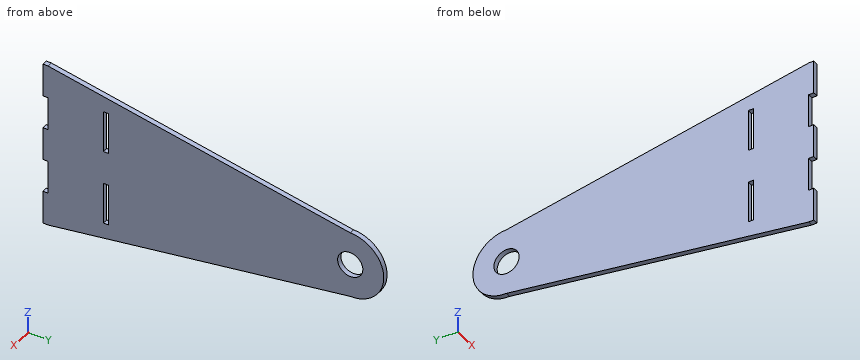
from build123d import *

# Parameters (mm, degrees)
SKETCH2_R           = 7.5
BOSS_EXTRUDE1_DEPTH = 1.5
SKETCH3_W           = 25
SKETCH3_H           = 3
CUT_EXTRUDE1_DEPTH  = 4
SKETCH4_W           = 3
SKETCH4_H           = 20
BOSS_EXTRUDE2_DEPTH = 3


with BuildPart() as part:
    # Sketch2 → Boss-Extrude1 (new, symmetric)
    with BuildSketch(Plane(origin=(0, 0, 0), x_dir=(0, 0, -1), z_dir=(1, 0, 0))):
        with BuildLine():
            Line((50, 0), (-50, 0))
            Line((-50, 0), (-20, 180))
            ThreePointArc((-20, 180), (0, 200), (20, 180))
            Line((20, 180), (50, 0))
        make_face()
        with Locations((0, 180)):
            Circle(SKETCH2_R, mode=Mode.SUBTRACT)
    extrude(amount=BOSS_EXTRUDE1_DEPTH, both=True)

    # Sketch3 → Cut-Extrude1 (cut)
    with BuildSketch(Plane.ZY.offset(1.5)):
        with Locations((22.5, 34.5)):
            Rectangle(SKETCH3_W, SKETCH3_H)
        with Locations((-22.5, 34.5)):
            Rectangle(SKETCH3_W, SKETCH3_H)
    extrude(amount=-CUT_EXTRUDE1_DEPTH, mode=Mode.SUBTRACT)

    # Sketch4 → Boss-Extrude2 (add)
    with BuildSketch(Plane.XZ):
        Rectangle(SKETCH4_W, SKETCH4_H)
        with Locations((0, -40)):
            Rectangle(SKETCH4_W, SKETCH4_H)
        with Locations((0, 40)):
            Rectangle(SKETCH4_W, SKETCH4_H)
    extrude(amount=BOSS_EXTRUDE2_DEPTH)


solid = part.part
Design review of the part built by this model. Coordinates are the model's own, in mm. Round coordinates to 2 decimals unless told otherwise and drop trailing zeros. Write each loop counter-clockwise with the first axis right and the second up, starting at its lowest first coordinate (ties: lowest second). Pieces come first, ordered by that corner, then holes. Notation, with made-up numbers: (46.25, 83.25) - (94.25, 83.25) arc R7 cw to (94.25, 88.25) - close; hole circle Ø1 at (-10.75, -31.75). An arc over 180 degrees is marked (long way). Return JSON: item names as keys, results as strings. Group by question number.
Item 1: We need section A-A on z = 0. Write out the cut boundary in (x, y).
Item 2: Insertion check: P1, Ø0.9, axis at x = 0.5, y = 34, coming from the +Z side; P2, Ø0.9, axis at x = -0.5, y = 34, coming from the -Z side; P3, Ø8, axis at y = 148, z = -29, coming from the -X side; P4, Ø1, axis at x = 0.5, y = 84.5, coming from the +Z side. Each pin has a flat end and moves straight along its axis. Give the tip position at first contact, or say it passes through.
Item 3: We need section B-B on x = 0. Write out the cut boundary in (y, z).
Item 4: We need section D-D on y = 49.5. Write out the cut boundary in (x, z).
Item 5: We need section C-C on z = 32. Write out the cut boundary in (x, y), and give its area (3 significant figures).
Item 6: For probe 1 along Y at (x, z) = (0.2, 0); probe 2 along Z at (x, y) = (0.25, 120); probe 3 along Y at (x, z) = (0.85, -5), list the stretches that pass through material, from the lowest coordinate up. Write a range as [from, to].
Model answer:
{
 "1": {"outline": "(-1.5, -3) - (1.5, -3) - (1.5, 172.5) - (-1.5, 172.5) - close; (-1.5, 187.5) - (1.5, 187.5) - (1.5, 200) - (-1.5, 200) - close"},
 "2": {"P1": "stops at z = 44.41", "P2": "stops at z = -44.41", "P3": "stops at x = -1.5", "P4": "stops at z = 36"},
 "3": {"outline": "(-3, -50) - (0, -50) - (180, -20) arc R20 ccw to (180, 20) - (0, 50) - (-3, 50) - (-3, 30) - (0, 30) - (0, 10) - (-3, 10) - (-3, -10) - (0, -10) - (0, -30) - (-3, -30) - close; hole (33, -35) - (36, -35) - (36, -10) - (33, -10) - close; hole (33, 10) - (36, 10) - (36, 35) - (33, 35) - close; hole circle Ø15 at (180, 0)"},
 "4": {"outline": "(-1.5, -41.75) - (1.5, -41.75) - (1.5, 41.75) - (-1.5, 41.75) - close"},
 "5": {"outline": "(-1.5, -3) - (1.5, -3) - (1.5, 33) - (-1.5, 33) - close; (-1.5, 36) - (1.5, 36) - (1.5, 108) - (-1.5, 108) - close", "area": "324 mm²"},
 "6": {"probe 1": "y = [-3, 172.5], [187.5, 200]", "probe 2": "z = [-30, 30]", "probe 3": "y = [-3, 174.41], [185.59, 199.36]"}
}
